from build123d import *

# Parameters (mm, degrees)
F1_DEPTH = 38.1
F3_DEPTH = 22.225
F4_R     = 14.351
F5_REACH = 121.9987572146
F6_R     = 12.6746
F7_DEPTH = 81.4079995473


# Not quite as in the source:
# - a feature names something its author has since deleted; it is built from what else it names


with BuildPart() as f1:
    # F0 (on Front) → F1 (new body, symmetric)
    with BuildSketch(Plane.XZ):
        with BuildLine():
            ThreePointArc((41.9913857052, 0), (37.8505272155, 1.5358758877), (35.7127694215, 5.4005382775))
            ThreePointArc((35.7127694215, 5.4005382775), (0, 36.1188), (-35.7127694215, 5.4005382775))
            ThreePointArc((-35.7127694215, 5.4005382775), (-37.8505272155, 1.5358758877), (-41.9913857052, 0))
            Line((-41.9913857052, 0), (-89.3826, 0))
            Line((-89.3826, 0), (-89.3826, -6.3499995473))
            Line((-89.3826, -6.3499995473), (-41.9913857052, -6.3499995473))
            ThreePointArc((-41.9913857052, -6.3499995473), (-33.7096690211, -3.2782478815), (-29.4341535854, 4.4510766227))
            ThreePointArc((-29.4341535854, 4.4510766227), (0, 29.7688004527), (29.4341535854, 4.4510766227))
            ThreePointArc((29.4341535854, 4.4510766227), (33.7096690211, -3.2782478815), (41.9913857052, -6.3499995473))
            Line((41.9913857052, -6.3499995473), (89.3826, -6.3499995473))
            Line((89.3826, -6.3499995473), (89.3826, 0))
            Line((89.3826, 0), (41.9913857052, 0))
        make_face()
    extrude(amount=F1_DEPTH, both=True)



with BuildPart() as f3:
    # F2 (on Front) → F3 (new body, symmetric)
    with BuildSketch(Plane.XZ):
        with BuildLine():
            Line((20.2057, 75.057), (0, 75.057))
            Line((0, 75.057), (-20.2057, 75.057))
            Line((-20.2057, 75.057), (-20.2057, 65.278))
            ThreePointArc((-20.2057, 65.278), (0, 61.6607352251), (20.2057, 65.278))
            Line((20.2057, 65.278), (20.2057, 75.057))
        make_face()
    extrude(amount=F3_DEPTH, both=True)


with BuildPart() as f1_1:
    add(f1.part)

    add(f3.part)  # F5 merges F3
    f5_end = f1_1.faces().sort_by_distance((0, 0, 36.1188))[0]
    # F4 (on face) → F5 (join, up to a face of the model that its end follows)
    with BuildSketch(Plane.XY.offset(75.057)):
        Circle(F4_R)
    f5_long = extrude(amount=-F5_REACH, mode=Mode.PRIVATE)
    add(split(f5_long, bisect_by=f5_end, keep=Keep.TOP, mode=Mode.PRIVATE))

    # F6 (on face) → F7 (cut, through all)
    with BuildSketch(Plane.XY.offset(75.057)):
        Circle(F6_R)
    extrude(amount=-F7_DEPTH, mode=Mode.SUBTRACT)


solid = f1_1.part
The listing builds one solid part. Answer for the finished solid, in the listing's coordinates (mm). A direction names the side the tool comes from. Round coordinates to 2 decimals unless told otherwise and drop trailing zeros. Write each loop counter-clockwise with the first axis right and the second up, starting at its lowest first coordinate (ties: lowest second). Pieces come first, ordered by that corner, then holes. Notation, with made-up numbers: M 1.5,54 L 46.5,54 A32 cw 46.5,87 Z; hole C 57,42.5 d7. An arc over 180 degrees is marked long. Write each question's results on one line, items separated by ' | '. Start each with the question number.
(1) Determine the mould class of faces 6 (the cylindrical face through (-9.8, -9, 28.11)), 7 (the flat face through (-65, -1, 0)), 8 (the flat face through (-89.383, -1, -3)) for opening direction X: +X half, -X half, draft (parallel to the pull), parting line (faces both ways), or undercut.
(2) The part is cut by section A-A, the plane y = 0. Write down the section's boundary in (x, z), and give its area (3 significant figures).
(3) The part is cut by section B-B, the plane x = 0. Write down the section's boundary in (y, z) (3 decimals), and give its area (3 significant figures).
(4) Each of these flat-tipped pins is pushed along its axis until it touches: P1, Ø5, axis at x = 24, y = -13.5, coming from the +Z side; P2, Ø23.5, axis at x = -71.5, y = -6, coming from the +Z side; P3, Ø2, axis at y = 7, z = 53, coming from the -X side; P4, Ø4, axis at x = -0.5, z = 37, coming from the -Y side. Where does it stop, or does it pass through?
(5) The part is cut by section D-D, the plane z = 59.5. Write down the section's boundary in (x, y).
(6) For faces 1 (the flat face through (0, 22.225, 68)), 2 (the cylindrical face through (-13.91, -5.25, 63.346)), 3 (the cylindrical face through (-33.806, -0.533, -3.36)), 4 (the flat face through (20.206, 0, 70)), 5 (the flat face through (-20.206, 0, 70)), determine the directions among +Z, -Z, +X, -X, +Y, -Y from which every point of the face is accessible in a straight line to the end or side of a thin tool.
(7) The part is cut by section C-C, the plane y = 29.5. Write down the section's boundary in (x, z).
(8) Find the intervals of material crossed by line 1 (X direction, y = 0, z = 61.5); line 2 (Z direction, x = 43, y = 17), in increasing order.
Worked answers:
1) face 6: undercut | face 7: draft | face 8: -X half
2) outline: M -89.38,-6.35 L -41.99,-6.35 A12.7 ccw -29.43,4.45 A29.77 cw -12.67,26.94 L -12.67,75.06 L -20.21,75.06 L -20.21,65.28 A58.24 ccw -14.35,63.46 L -14.35,33.15 A36.12 ccw -35.71,5.4 A6.35 cw -41.99,0 L -89.38,0 Z; M 12.67,26.94 A29.77 cw 29.43,4.45 A12.7 ccw 41.99,-6.35 L 89.38,-6.35 L 89.38,0 L 41.99,0 A6.35 cw 35.71,5.4 A36.12 ccw 14.35,33.15 L 14.35,63.46 A58.24 ccw 20.21,65.28 L 20.21,75.06 L 12.67,75.06 Z | area: 1,470 mm²
3) outline: M -38.1,29.769 L -12.675,29.769 L -12.675,75.057 L -22.225,75.057 L -22.225,61.661 L -14.351,61.661 L -14.351,36.119 L -38.1,36.119 Z; M 12.675,29.769 L 38.1,29.769 L 38.1,36.119 L 14.351,36.119 L 14.351,61.661 L 22.225,61.661 L 22.225,75.057 L 12.675,75.057 Z | area: 664 mm²
4) P1: stops at z = 29.02 | P2: stops at z = 0 | P3: stops at x = -13.04 | P4: stops at y = -38.1
5) outline: C 0,0 d28.7; hole C 0,0 d25.35
6) face 1: +Z, +X, -X, +Y | face 2: none | face 3: -Z, +Y, -Y | face 4: +Z, +X, +Y, -Y | face 5: +Z, -X, +Y, -Y
7) outline: M -89.38,-6.35 L -41.99,-6.35 A12.7 ccw -29.43,4.45 A29.77 cw 29.43,4.45 A12.7 ccw 41.99,-6.35 L 89.38,-6.35 L 89.38,0 L 41.99,0 A6.35 cw 35.71,5.4 A36.12 ccw -35.71,5.4 A6.35 cw -41.99,0 L -89.38,0 Z
8) line 1: x = -14.35 to -12.67, 12.67 to 14.35 | line 2: z = -6.35 to 0
